Verification items for the finished model (mm, model axes). Face numbers are marked on the shaded views. A direction names the side the tool comes from. Round coordinates to 2 decimals unless told otherwise and drop trailing zeros. Write each loop counter-clockwise with the first axis right and the second up, starting at its lowest first coordinate (ties: lowest second). Pieces come first, ordered by that corner, then holes. Notation, with made-up numbers: (39, 64) - (93, 64) arc R22 cw to (93, 85) - close; hole circle Ø6 at (-25.5, 59). An arc over 180 degrees is marked (long way). Write each question's results on one line, items separated by ' | '.
```python
from build123d import *

# Parameters (mm, degrees)
BOSS_EXTRUDE1_DEPTH      = 4.5
CUT_EXTRUDE3_DEPTH       = 2.1
BOSS_EXTRUDE3_START      = 6.5
BOSS_EXTRUDE3_DEPTH      = 6.5
CUT_EXTRUDE4_START       = 4.1
CUT_EXTRUDE4_DEPTH       = 4.1
BOSS_EXTRUDE4_DEPTH      = 3
BOSS_EXTRUDE4_DEPTH_BACK = 3
SKETCH4_R                = 1.25
SKETCH4_W                = 6
SKETCH4_H                = 8
FILLET1_R                = 1.5
SKETCH5_W                = 150
SKETCH5_H                = 40
CUT_EXTRUDE5_DEPTH       = 79.451654949


with BuildPart() as part:
    # Sketch2 → Boss-Extrude1 (new body)
    with BuildSketch(Plane(origin=(0, 0, 0), x_dir=(1, 0, 0), z_dir=(0, 1, 0))):
        with BuildLine():
            Line((-28.15, 50), (28.15, 50))
            ThreePointArc((28.15, 50), (35.221067812, 47.071067812), (38.15, 40))
            Line((38.15, 40), (38.15, 18.869079534))
            Line((38.15, 18.869079534), (37.959241868, 14.5))
            Line((37.959241868, 14.5), (50.123967842, 14.5))
            Line((50.123967842, 14.5), (50.123967842, -10.5))
            Line((50.123967842, -10.5), (35.7933894, -10.5))
            Line((35.7933894, -10.5), (29.904245688, -43.067652969))
            ThreePointArc((29.904245688, -43.067652969), (28.715879749, -46.302425464), (26.5, -48.941713937))
            Line((26.5, -48.941713937), (26.5, -52.373001444))
            ThreePointArc((26.5, -52.373001444), (0, -54), (-26.5, -52.373001444))
            Line((-26.5, -52.373001444), (-26.5, -48.941713937))
            ThreePointArc((-26.5, -48.941713937), (-28.715879749, -46.302425464), (-29.904245688, -43.067652969))
            Line((-29.904245688, -43.067652969), (-35.7933894, -10.5))
            Line((-35.7933894, -10.5), (-50.123967842, -10.5))
            Line((-50.123967842, -10.5), (-50.123967842, 14.5))
            Line((-50.123967842, 14.5), (-37.959241868, 14.5))
            Line((-37.959241868, 14.5), (-38.15, 18.869079534))
            Line((-38.15, 18.869079534), (-38.15, 40))
            ThreePointArc((-38.15, 40), (-35.221067812, 47.071067812), (-28.15, 50))
        make_face()
        with BuildLine():
            Line((-32.75, 40), (-32.75, 18.986907953))
            Line((-32.75, 18.986907953), (-32.318328276, 9.1))
            Line((-32.318328276, 9.1), (-44.723967842, 9.1))
            Line((-44.723967842, 9.1), (-44.723967842, -5.1))
            Line((-44.723967842, -5.1), (-31.282284108, -5.1))
            Line((-31.282284108, -5.1), (-24.590424569, -42.106765297))
            ThreePointArc((-24.590424569, -42.106765297), (-23.494161062, -44.35301053), (-21.385106897, -45.694391107))
            ThreePointArc((-21.385106897, -45.694391107), (-21.179097179, -45.838743936), (-21.1, -46.077535434))
            Line((-21.1, -46.077535434), (-21.1, -47.543481521))
            ThreePointArc((-21.1, -47.543481521), (0, -48.6), (21.1, -47.543481521))
            Line((21.1, -47.543481521), (21.1, -46.077535434))
            ThreePointArc((21.1, -46.077535434), (21.179097179, -45.838743936), (21.385106897, -45.694391107))
            ThreePointArc((21.385106897, -45.694391107), (23.494161062, -44.35301053), (24.590424569, -42.106765297))
            Line((24.590424569, -42.106765297), (31.282284108, -5.1))
            Line((31.282284108, -5.1), (44.723967842, -5.1))
            Line((44.723967842, -5.1), (44.723967842, 9.1))
            Line((44.723967842, 9.1), (32.318328276, 9.1))
            Line((32.318328276, 9.1), (32.75, 18.986907953))
            Line((32.75, 18.986907953), (32.75, 40))
            ThreePointArc((32.75, 40), (31.402691193, 43.252691193), (28.15, 44.6))
            Line((28.15, 44.6), (-28.15, 44.6))
            ThreePointArc((-28.15, 44.6), (-31.402691193, 43.252691193), (-32.75, 40))
        make_face(mode=Mode.SUBTRACT)
    extrude(amount=-BOSS_EXTRUDE1_DEPTH)

    # Sketch2<6> → Cut-Extrude3 (cut)
    with BuildSketch(Plane(origin=(0, 0, 0), x_dir=(1, 0, 0), z_dir=(0, 1, 0))):
        with BuildLine():
            Line((-28.15, 46.7), (28.15, 46.7))
            ThreePointArc((28.15, 46.7), (32.887615434, 44.737615434), (34.85, 40))
            Line((34.85, 40), (34.85, 18.94108579))
            Line((34.85, 18.94108579), (34.512016895, 11.2))
            Line((34.512016895, 11.2), (46.823967842, 11.2))
            Line((46.823967842, 11.2), (46.823967842, -7.2))
            Line((46.823967842, -7.2), (33.036602833, -7.2))
            Line((33.036602833, -7.2), (26.656910559, -42.480443836))
            ThreePointArc((26.656910559, -42.480443836), (25.472544462, -45.242453785), (23.2, -47.208913466))
            Line((23.2, -47.208913466), (23.2, -49.434698257))
            ThreePointArc((23.2, -49.434698257), (0, -50.7), (-23.2, -49.434698257))
            Line((-23.2, -49.434698257), (-23.2, -47.208913466))
            ThreePointArc((-23.2, -47.208913466), (-25.472544462, -45.242453785), (-26.656910559, -42.480443836))
            Line((-26.656910559, -42.480443836), (-33.036602833, -7.2))
            Line((-33.036602833, -7.2), (-46.823967842, -7.2))
            Line((-46.823967842, -7.2), (-46.823967842, 11.2))
            Line((-46.823967842, 11.2), (-34.512016895, 11.2))
            Line((-34.512016895, 11.2), (-34.85, 18.94108579))
            Line((-34.85, 18.94108579), (-34.85, 40))
            ThreePointArc((-34.85, 40), (-32.887615434, 44.737615434), (-28.15, 46.7))
        make_face()
    extrude(amount=-CUT_EXTRUDE3_DEPTH, mode=Mode.SUBTRACT)

    # Sketch2<7> → Boss-Extrude3 (add)
    with BuildSketch(Plane(origin=(0, 0, 0), x_dir=(1, 0, 0), z_dir=(0, 1, 0)).offset(BOSS_EXTRUDE3_START)):
        with BuildLine():
            Line((28.15, 50), (-28.15, 50))
            ThreePointArc((-28.15, 50), (-35.221067812, 47.071067812), (-38.15, 40))
            Line((-38.15, 40), (-38.15, 18.869079534))
            Line((-38.15, 18.869079534), (-37.959241868, 14.5))
            Line((-37.959241868, 14.5), (-50.123967842, 14.5))
            Line((-50.123967842, 14.5), (-50.123967842, -10.5))
            Line((-50.123967842, -10.5), (-35.7933894, -10.5))
            Line((-35.7933894, -10.5), (-29.904245688, -43.067652969))
            ThreePointArc((-29.904245688, -43.067652969), (-28.715879749, -46.302425464), (-26.5, -48.941713937))
            Line((-26.5, -48.941713937), (-26.5, -52.373001444))
            ThreePointArc((-26.5, -52.373001444), (0, -54), (26.5, -52.373001444))
            Line((26.5, -52.373001444), (26.5, -48.941713937))
            ThreePointArc((26.5, -48.941713937), (28.715879749, -46.302425464), (29.904245688, -43.067652969))
            Line((29.904245688, -43.067652969), (35.7933894, -10.5))
            Line((35.7933894, -10.5), (50.123967842, -10.5))
            Line((50.123967842, -10.5), (50.123967842, 14.5))
            Line((50.123967842, 14.5), (37.959241868, 14.5))
            Line((37.959241868, 14.5), (38.15, 18.869079534))
            Line((38.15, 18.869079534), (38.15, 40))
            ThreePointArc((38.15, 40), (35.221067812, 47.071067812), (28.15, 50))
        make_face()
        with BuildLine():
            Line((-44.723967842, 9.1), (-32.318328276, 9.1))
            Line((-32.318328276, 9.1), (-32.75, 18.986907953))
            Line((-32.75, 18.986907953), (-32.75, 40))
            ThreePointArc((-32.75, 40), (-31.402691193, 43.252691193), (-28.15, 44.6))
            Line((-28.15, 44.6), (28.15, 44.6))
            ThreePointArc((28.15, 44.6), (31.402691193, 43.252691193), (32.75, 40))
            Line((32.75, 40), (32.75, 18.986907953))
            Line((32.75, 18.986907953), (32.318328276, 9.1))
            Line((32.318328276, 9.1), (44.723967842, 9.1))
            Line((44.723967842, 9.1), (44.723967842, -5.1))
            Line((44.723967842, -5.1), (31.282284108, -5.1))
            Line((31.282284108, -5.1), (24.590424569, -42.106765297))
            ThreePointArc((24.590424569, -42.106765297), (23.494161062, -44.35301053), (21.385106897, -45.694391107))
            ThreePointArc((21.385106897, -45.694391107), (21.179097179, -45.838743936), (21.1, -46.077535434))
            Line((21.1, -46.077535434), (21.1, -47.543481521))
            ThreePointArc((21.1, -47.543481521), (0, -48.6), (-21.1, -47.543481521))
            Line((-21.1, -47.543481521), (-21.1, -46.077535434))
            ThreePointArc((-21.1, -46.077535434), (-21.179097179, -45.838743936), (-21.385106897, -45.694391107))
            ThreePointArc((-21.385106897, -45.694391107), (-23.494161062, -44.35301053), (-24.590424569, -42.106765297))
            Line((-24.590424569, -42.106765297), (-31.282284108, -5.1))
            Line((-31.282284108, -5.1), (-44.723967842, -5.1))
            Line((-44.723967842, -5.1), (-44.723967842, 9.1))
        make_face(mode=Mode.SUBTRACT)
    extrude(amount=-BOSS_EXTRUDE3_DEPTH)

    # Sketch2<8> → Cut-Extrude4 (cut)
    with BuildSketch(Plane(origin=(0, 0, 0), x_dir=(1, 0, 0), z_dir=(0, 1, 0)).offset(CUT_EXTRUDE4_START)):
        with BuildLine():
            Line((28.15, 46.7), (-28.15, 46.7))
            ThreePointArc((-28.15, 46.7), (-32.887615434, 44.737615434), (-34.85, 40))
            Line((-34.85, 40), (-34.85, 18.94108579))
            Line((-34.85, 18.94108579), (-34.512016895, 11.2))
            Line((-34.512016895, 11.2), (-46.823967842, 11.2))
            Line((-46.823967842, 11.2), (-46.823967842, -7.2))
            Line((-46.823967842, -7.2), (-33.036602833, -7.2))
            Line((-33.036602833, -7.2), (-26.656910559, -42.480443836))
            ThreePointArc((-26.656910559, -42.480443836), (-25.472544462, -45.242453785), (-23.2, -47.208913466))
            Line((-23.2, -47.208913466), (-23.2, -49.434698257))
            ThreePointArc((-23.2, -49.434698257), (0, -50.7), (23.2, -49.434698257))
            Line((23.2, -49.434698257), (23.2, -47.208913466))
            ThreePointArc((23.2, -47.208913466), (25.472544462, -45.242453785), (26.656910559, -42.480443836))
            Line((26.656910559, -42.480443836), (33.036602833, -7.2))
            Line((33.036602833, -7.2), (46.823967842, -7.2))
            Line((46.823967842, -7.2), (46.823967842, 11.2))
            Line((46.823967842, 11.2), (34.512016895, 11.2))
            Line((34.512016895, 11.2), (34.85, 18.94108579))
            Line((34.85, 18.94108579), (34.85, 40))
            ThreePointArc((34.85, 40), (32.887615434, 44.737615434), (28.15, 46.7))
        make_face()
        with BuildLine():
            Line((-32.75, 18.986907953), (-32.75, 40))
            ThreePointArc((-32.75, 40), (-31.402691193, 43.252691193), (-28.15, 44.6))
            Line((-28.15, 44.6), (28.15, 44.6))
            ThreePointArc((28.15, 44.6), (31.402691193, 43.252691193), (32.75, 40))
            Line((32.75, 40), (32.75, 18.986907953))
            Line((32.75, 18.986907953), (32.318328276, 9.1))
            Line((32.318328276, 9.1), (44.723967842, 9.1))
            Line((44.723967842, 9.1), (44.723967842, -5.1))
            Line((44.723967842, -5.1), (31.282284108, -5.1))
            Line((31.282284108, -5.1), (24.590424569, -42.106765297))
            ThreePointArc((24.590424569, -42.106765297), (23.494161062, -44.35301053), (21.385106897, -45.694391107))
            ThreePointArc((21.385106897, -45.694391107), (21.179097179, -45.838743936), (21.1, -46.077535434))
            Line((21.1, -46.077535434), (21.1, -47.543481521))
            ThreePointArc((21.1, -47.543481521), (0, -48.6), (-21.1, -47.543481521))
            Line((-21.1, -47.543481521), (-21.1, -46.077535434))
            ThreePointArc((-21.1, -46.077535434), (-21.179097179, -45.838743936), (-21.385106897, -45.694391107))
            ThreePointArc((-21.385106897, -45.694391107), (-23.494161062, -44.35301053), (-24.590424569, -42.106765297))
            Line((-24.590424569, -42.106765297), (-31.282284108, -5.1))
            Line((-31.282284108, -5.1), (-44.723967842, -5.1))
            Line((-44.723967842, -5.1), (-44.723967842, 9.1))
            Line((-44.723967842, 9.1), (-32.318328276, 9.1))
            Line((-32.318328276, 9.1), (-32.75, 18.986907953))
        make_face(mode=Mode.SUBTRACT)
    extrude(amount=-CUT_EXTRUDE4_DEPTH, mode=Mode.SUBTRACT)

    # Sketch4 → Boss-Extrude4 (add, two sides: drawn at the far end of the back side and taken through both)
    # profile 1 of 2: a face of its own
    with BuildSketch(Plane(origin=(0, 0, 0), x_dir=(0, 0, -1), z_dir=(1, 0, 0)).offset(-BOSS_EXTRUDE4_DEPTH_BACK)):
        Polygon((-52, 5), (-52, -3), (-54, -3), (-60, -3), (-60, 5), (-54, 5), align=None)
        with Locations((-57, 1)):
            Circle(SKETCH4_R, mode=Mode.SUBTRACT)
    # profile 2 of 2: a face of its own
    with BuildSketch(Plane(origin=(0, 0, 0), x_dir=(0, 0, -1), z_dir=(1, 0, 0)).offset(-BOSS_EXTRUDE4_DEPTH_BACK)):
        with Locations((53, 1)):
            Rectangle(SKETCH4_W, SKETCH4_H)
        with Locations((53, 1)):
            Circle(SKETCH4_R, mode=Mode.SUBTRACT)
    extrude(amount=BOSS_EXTRUDE4_DEPTH + BOSS_EXTRUDE4_DEPTH_BACK)

    # Fillet1
    fillet1_edges = [part.edges().sort_by_distance(p)[0] for p in [
        (0, 5, 54),
        (0, -3, 54),
        (0, -3, -50),
        (0, 5, -50),
    ]]
    fillet(fillet1_edges, radius=FILLET1_R - 0.0001)  # a hair under: the kernel refuses the full size

    # Sketch5 → Cut-Extrude5 (cut, through all)
    with BuildSketch(Plane(origin=(0, 0, 0), x_dir=(0, 0, -1), z_dir=(1, 0, 0))):
        Rectangle(SKETCH5_W, SKETCH5_H)
    extrude(amount=-CUT_EXTRUDE5_DEPTH, mode=Mode.SUBTRACT)


solid = part.part
```
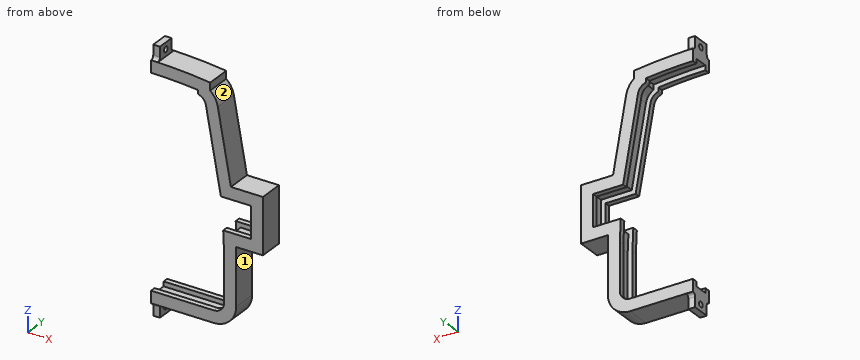
(1) Section check B-B (x = 40). Record the cut outline in (y, z), plus the area to 3 significant figures.
Answer:
outline: (-4.5, -14.5) - (6.5, -14.5) - (6.5, -9.1) - (4.1, -9.1) - (4.1, -11.2) - (-2.1, -11.2) - (-2.1, -9.1) - (-4.5, -9.1) - close; (-4.5, 5.1) - (-2.1, 5.1) - (-2.1, 7.2) - (4.1, 7.2) - (4.1, 5.1) - (6.5, 5.1) - (6.5, 10.5) - (-4.5, 10.5) - close | area: 92.8 mm2
(2) Section check C-C (z = -35). Record the cut outline in (x, y).
Answer:
outline: (32.75, -4.5) - (38.15, -4.5) - (38.15, 6.5) - (32.75, 6.5) - (32.75, 4.1) - (34.85, 4.1) - (34.85, -2.1) - (32.75, -2.1) - close
(3) Section check D-D (y = 1). State how many separate pieces and enclosed holes the cut face has, plus the area to 3 significant figures.
Answer:
separate pieces: 3 | enclosed holes: 0 | area: 632 mm2
(4) Thickness scan on L1, parallel to Z at x = 1.75, y = 1; L2, parallel to Y at x = 2, z = -53; L3, parallel to Z at x = 2, y = 2.5. Record the ranges inside material, lowest first.
Answer:
L1: -56 to -54.25, -51.75 to -46.7, 50.69 to 55.75, 58.25 to 60 | L2: -3 to -0.25, 2.25 to 5 | L3: -56 to -46.7, 50.69 to 60
(5) Section check A-A (z = -53). Record the cut outline in (x, y).
Answer:
outline: (0, -3) - (3, -3) - (3, -0.25) - (0, -0.25) - close; (0, 2.25) - (3, 2.25) - (3, 5) - (0, 5) - close
(6) Go/stop test with flat-tipped pins: pin 1 Ø1.5 at (x, y) = (31.5, 2.5) entering from -Z; pin 2 Ø3 at (x, y) = (29, 3) entering from -Z; pin 3 Ø2.5 at (x, z) = (1.5, -55) entering from +Y. Record where each tip stops, or that it passes through.
Answer:
pin 1: z = -49.66 | pin 2: z = -50 | pin 3: y = 5
(7) Set-up check for the marked faces 1 and 2: record each of +Z, -Z, +X, -X, +Y, -Y from which the full face is reachable in a straight line by a thin tool's end or side.
Answer:
face 1: -Z, +X, +Y, -Y | face 2: +Z, +X, +Y, -Y
